Can you work these out from the model? Positions are in its coordinate system, mm. Face numbers are marked on the shaded views. A direction names the side the tool comes from. Round coordinates to 2 decimals unless told otherwise and drop trailing zeros. Order: outer loops, then holes, each group sorted by start corner. A loop starts at its lowest first (then second) coordinate and runs counter-clockwise, first axis right, second up.
Q1. Will these pins go through, and if not, where does the flat tip stop? P1, Ø12, axis at x = 12.5, y = 60, coming from the -Z side; P2, Ø3, axis at x = -19, y = 40, coming from the +Z side; P3, Ø6, axis at y = 86.5, z = 5.1, coming from the +X side; P4, Ø1.2, axis at y = 67, z = 11.5, coming from the -X side.
Q2. We'd pull the mould along Z, two halves only. Please class the marked faces 4, 5 and 6: pulls with the +Z half, pulls with the -Z half, needs draft (parallel to the pull), parting line crosses it, or undercut.
Q3. For the marked faces 1, 2 and 3, which set-ups out of +Z, -Z, +X, -X, +Y, -Y let a thin tool reach every point of the face, with its end or its side?
Q4. If I drill on line 1 (Y direction, x = 1.9, z = 5.1); line 2 (Z direction, x = 4, y = 47.5); line 3 (Y direction, x = 21.5, z = -4), over which ranges is the centre line in solid material (lowest first)?
Q5. If we section it at C-C (y = 62): Please give me the cut outline in (x, z), plus the area to 3 significant figures.
Q6. If we section it at A-A (y = 86.5): Please give me the cut outline in (x, z), plus the area to 3 significant figures.
Q7. If we section it at B-B (z = -5.1): Count the separate pieces of the cut face and the enclosed holes in it, plus the area to 3 significant figures.
from build123d import *

# Parameters (mm, degrees)
SKETCH1_W           = 3
SKETCH1_H           = 4
SKETCH1_W_2         = 25
SKETCH1_H_2         = 35
SKETCH2_W           = 4.909608088
SKETCH2_H           = 2.5
SKETCH2_W_2         = 1
BOSS_EXTRUDE1_DEPTH = 55
CHAMFER1_SIZE       = 10
CHAMFER1_SIZE2      = 30
CHAMFER2_SIZE       = 20
SKETCH3_R           = 2.25
SKETCH3_W           = 20
SKETCH3_H           = 41.913950128
SKETCH3_W_2         = 1.5
SKETCH3_H_2         = 5.443024936
SKETCH3_W_3         = 1.501012669
CUT_EXTRUDE1_DEPTH  = 55
SKETCH5_W           = 15.682680147
SKETCH5_H           = 21
CUT_EXTRUDE2_DEPTH  = 36


with BuildPart() as part:
    # Sketch1 → Revolve1 (revolve)
    with BuildSketch(Plane.XY):
        with Locations((26.5, 12.5)):
            Rectangle(SKETCH1_W, SKETCH1_H)
        with Locations((12.5, 17.5)):
            Rectangle(SKETCH1_W_2, SKETCH1_H_2)
    revolve(axis=Axis((0, 35, 0), (0, -1, 0)))

    # Sketch2 → Boss-Extrude1 (add)
    with BuildSketch(Plane(origin=(0, 35, 0), x_dir=(1, 0, 0), z_dir=(0, 1, 0))):
        Polygon((4.5, 10.5), (4.5, 13), (0, 13), (0, 10.5), (0, -10.5), (0, -13), (4.5, -13), (4.5, -10.5), align=None)
        with Locations((6.954804044, 11.75)):
            Rectangle(SKETCH2_W, SKETCH2_H)
        with Locations((6.954804044, -11.75)):
            Rectangle(SKETCH2_W, SKETCH2_H)
        with Locations((-0.5, -11.75)):
            Rectangle(SKETCH2_W_2, SKETCH2_H)
        with Locations((-0.5, 11.75)):
            Rectangle(SKETCH2_W_2, SKETCH2_H)
    extrude(amount=BOSS_EXTRUDE1_DEPTH)

    # Chamfer1
    chamfer1_edges = [part.edges().sort_by_distance(p)[0] for p in [
        (9.409608088, 35, 11.75),
        (9.409608088, 35, -11.75),
    ]]
    chamfer1_side = [part.faces().sort_by_distance(p)[0] for p in [
        (-0.237473478, 35, 0),
    ]]
    chamfer(chamfer1_edges, length=CHAMFER1_SIZE, length2=CHAMFER1_SIZE2, reference=chamfer1_side[0])

    # Chamfer2
    chamfer2_edges = [part.edges().sort_by_distance(p)[0] for p in [
        (-1, 35, -11.75),
        (-1, 35, 11.75),
    ]]
    chamfer(chamfer2_edges, length=CHAMFER2_SIZE)

    # Sketch3 → Cut-Extrude1 (cut)
    with BuildSketch(Plane(origin=(4.5, 0, 0), x_dir=(0, 0, -1), z_dir=(1, 0, 0))):
        with Locations((-5.1, 86.5)):
            Circle(SKETCH3_R)
        with Locations((5.1, 86.5)):
            Circle(SKETCH3_R)
        with Locations((-5.1, 38.7)):
            Circle(SKETCH3_R)
        with Locations((5.1, 38.7)):
            Circle(SKETCH3_R)
        with Locations((0, 62.6)):
            Rectangle(SKETCH3_W, SKETCH3_H)
        with Locations((0, 86.278487532)):
            Rectangle(SKETCH3_W_2, SKETCH3_H_2)
        with Locations((-0.000506335, 38.921512468)):
            Rectangle(SKETCH3_W_3, SKETCH3_H_2)
    extrude(amount=-CUT_EXTRUDE1_DEPTH, mode=Mode.SUBTRACT)

    # Sketch5 → Cut-Extrude2 (cut, through all)
    with BuildSketch(Plane(origin=(0, 35, 0), x_dir=(1, 0, 0), z_dir=(0, 1, 0))):
        with Locations((-7.841340074, 0)):
            Rectangle(SKETCH5_W, SKETCH5_H)
    extrude(amount=-CUT_EXTRUDE2_DEPTH, mode=Mode.SUBTRACT)


solid = part.part
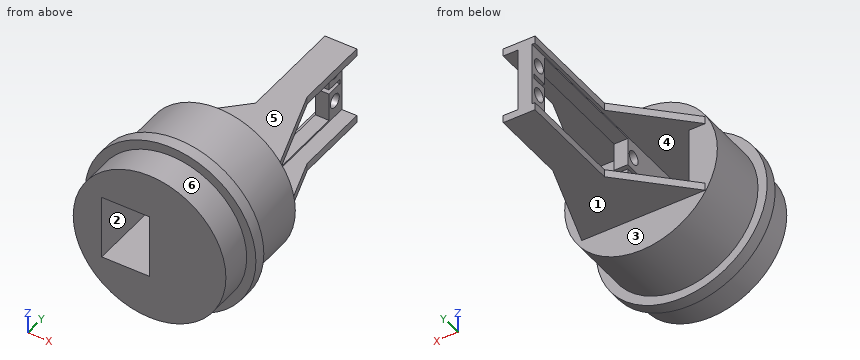
Solution:
1. P1: stops at z = -13
1. P2: passes through
1. P3: stops at x = 4.5
1. P4: stops at x = -1
2. face 4: undercut
2. face 5: pulls with the +Z half
2. face 6: parting line crosses it
3. face 1: -Z, +X, -X, +Y
3. face 2: +Y, -Y
3. face 3: +Y
4. line 1: y = 0 to 36.45, 40.95 to 41.64, 83.56 to 84.25, 88.75 to 90
4. line 2: z = -13 to -10, 10 to 13
4. line 3: y = 0 to 35
5. outline: (-1, -13) - (10.41, -13) - (10.41, -10.5) - (4.5, -10.5) - (4.5, -10) - (0, -10) - (0, -10.5) - (-1, -10.5) - close; (-1, 10.5) - (0, 10.5) - (0, 10) - (4.5, 10) - (4.5, 10.5) - (10.41, 10.5) - (10.41, 13) - (-1, 13) - close
5. area: 61.5 mm2
6. outline: (-1, -13) - (9.41, -13) - (9.41, -10.5) - (4.5, -10.5) - (4.5, -7.35) - (0, -7.35) - (0, -10.5) - (-1, -10.5) - close; (-1, 10.5) - (0, 10.5) - (0, 7.35) - (4.5, 7.35) - (4.5, 10.5) - (9.41, 10.5) - (9.41, 13) - (-1, 13) - close; (0, -2.85) - (4.5, -2.85) - (4.5, -0.75) - (0, -0.75) - close; (0, 0.75) - (4.5, 0.75) - (4.5, 2.85) - (0, 2.85) - close
6. area: 99.3 mm2
7. separate pieces: 5
7. enclosed holes: 0
7. area: 1,210 mm2
